from build123d import *

# Parameters (mm, degrees)
F1_DEPTH    = 80
F0_R        = 10
F2_DEPTH    = 40
F0_R_2      = 4
F3_DEPTH    = 5
F4_SIZE     = 2
F5_T1_DEPTH = 43.847334297


# Not quite as in the source:
# - a fillet or chamfer that OpenCascade refuses, or shapes differently, is made with other operations: its cross-section is extruded or revolved along the edge and cut away or added


with BuildPart() as f1:
    # F0 (on Top) → F1 (new body)
    with BuildSketch(Plane.XY):
        with BuildLine():
            ThreePointArc((26.9229627936, -13.2345787395), (29.220616727, -6.7937881992), (30, 0))
            ThreePointArc((30, 0), (29.220616727, 6.7937881992), (26.9229627936, 13.2345787395))
            Line((26.9229627936, 13.2345787395), (18.2336879396, 8.2178235635))
            ThreePointArc((18.2336879396, 8.2178235635), (19.5534365112, 4.2027515515), (20, 0))
            ThreePointArc((20, 0), (19.5534365112, -4.2027515515), (18.2336879396, -8.2178235635))
            Line((18.2336879396, -8.2178235635), (26.9229627936, -13.2345787395))
        make_face()
    extrude(amount=F1_DEPTH)



with BuildPart() as f1b:
    # F0 (on Top) → F1, piece 2 (new body)
    with BuildSketch(Plane.XY):
        with BuildLine():
            Line((16.2336879396, 11.6819251786), (24.9229627936, 16.6986803547))
            ThreePointArc((24.9229627936, 16.6986803547), (15.21659411, 25.8545018071), (2.5, 29.8956518578))
            Line((2.5, 29.8956518578), (2.5, 19.843134833))
            ThreePointArc((2.5, 19.843134833), (10.2170984976, 17.1933387767), (16.2336879396, 11.6819251786))
        make_face()
    extrude(amount=F1_DEPTH)


with BuildPart() as f1c:
    # F0 (on Top) → F1, piece 3 (new body)
    with BuildSketch(Plane.XY):
        with BuildLine():
            ThreePointArc((2.5, -29.8956518578), (15.21659411, -25.8545018071), (24.9229627936, -16.6986803547))
            Line((24.9229627936, -16.6986803547), (16.2336879396, -11.6819251786))
            ThreePointArc((16.2336879396, -11.6819251786), (10.2170984976, -17.1933387767), (2.5, -19.843134833))
            Line((2.5, -19.843134833), (2.5, -29.8956518578))
        make_face()
    extrude(amount=F1_DEPTH)


with BuildPart() as f1d:
    # F0 (on Top) → F1, piece 4 (new body)
    with BuildSketch(Plane.XY):
        with BuildLine():
            Line((-2.5, 19.843134833), (-2.5, 29.8956518578))
            ThreePointArc((-2.5, 29.8956518578), (-15.21659411, 25.8545018071), (-24.9229627936, 16.6986803547))
            Line((-24.9229627936, 16.6986803547), (-16.2336879396, 11.6819251786))
            ThreePointArc((-16.2336879396, 11.6819251786), (-10.2170984976, 17.1933387767), (-2.5, 19.843134833))
        make_face()
    extrude(amount=F1_DEPTH)


with BuildPart() as f1e:
    # F0 (on Top) → F1, piece 5 (new body)
    with BuildSketch(Plane.XY):
        with BuildLine():
            ThreePointArc((-24.9229627936, -16.6986803547), (-15.21659411, -25.8545018071), (-2.5, -29.8956518578))
            Line((-2.5, -29.8956518578), (-2.5, -19.843134833))
            ThreePointArc((-2.5, -19.843134833), (-10.2170984976, -17.1933387767), (-16.2336879396, -11.6819251786))
            Line((-16.2336879396, -11.6819251786), (-24.9229627936, -16.6986803547))
        make_face()
    extrude(amount=F1_DEPTH)


with BuildPart() as f1f:
    # F0 (on Top) → F1, piece 6 (new body)
    with BuildSketch(Plane.XY):
        with BuildLine():
            Line((-18.2336879396, 8.2178235635), (-26.9229627936, 13.2345787395))
            ThreePointArc((-26.9229627936, 13.2345787395), (-30, 0), (-26.9229627936, -13.2345787395))
            Line((-26.9229627936, -13.2345787395), (-18.2336879396, -8.2178235635))
            ThreePointArc((-18.2336879396, -8.2178235635), (-20, 0), (-18.2336879396, 8.2178235635))
        make_face()
    extrude(amount=F1_DEPTH)


with BuildPart() as f1_1:
    add(f1.part)

    add(f1b.part)  # F2 merges F1b

    add(f1c.part)  # F2 merges F1c

    add(f1d.part)  # F2 merges F1d

    add(f1e.part)  # F2 merges F1e

    add(f1f.part)  # F2 merges F1f
    # F0 (on Top) → F2 (join)
    with BuildSketch(Plane.XY):
        with BuildLine():
            Line((18.2336879396, 8.2178235635), (26.9229627936, 13.2345787395))
            ThreePointArc((26.9229627936, 13.2345787395), (25.9807621135, 15), (24.9229627936, 16.6986803547))
            Line((24.9229627936, 16.6986803547), (16.2336879396, 11.6819251786))
            ThreePointArc((16.2336879396, 11.6819251786), (17.3205080757, 10), (18.2336879396, 8.2178235635))
        make_face()
        with BuildLine():
            ThreePointArc((24.9229627936, -16.6986803547), (25.9807621135, -15), (26.9229627936, -13.2345787395))
            Line((26.9229627936, -13.2345787395), (18.2336879396, -8.2178235635))
            ThreePointArc((18.2336879396, -8.2178235635), (17.3205080757, -10), (16.2336879396, -11.6819251786))
            Line((16.2336879396, -11.6819251786), (24.9229627936, -16.6986803547))
        make_face()
        with BuildLine():
            ThreePointArc((20, 0), (19.5534365112, 4.2027515515), (18.2336879396, 8.2178235635))
            ThreePointArc((18.2336879396, 8.2178235635), (17.3205080757, 10), (16.2336879396, 11.6819251786))
            ThreePointArc((16.2336879396, 11.6819251786), (10.2170984976, 17.1933387767), (2.5, 19.843134833))
            ThreePointArc((2.5, 19.843134833), (0, 20), (-2.5, 19.843134833))
            ThreePointArc((-2.5, 19.843134833), (-10.2170984976, 17.1933387767), (-16.2336879396, 11.6819251786))
            ThreePointArc((-16.2336879396, 11.6819251786), (-17.3205080757, 10), (-18.2336879396, 8.2178235635))
            ThreePointArc((-18.2336879396, 8.2178235635), (-20, 0), (-18.2336879396, -8.2178235635))
            ThreePointArc((-18.2336879396, -8.2178235635), (-17.3205080757, -10), (-16.2336879396, -11.6819251786))
            ThreePointArc((-16.2336879396, -11.6819251786), (-10.2170984976, -17.1933387767), (-2.5, -19.843134833))
            ThreePointArc((-2.5, -19.843134833), (0, -20), (2.5, -19.843134833))
            ThreePointArc((2.5, -19.843134833), (10.2170984976, -17.1933387767), (16.2336879396, -11.6819251786))
            ThreePointArc((16.2336879396, -11.6819251786), (17.3205080757, -10), (18.2336879396, -8.2178235635))
            ThreePointArc((18.2336879396, -8.2178235635), (19.5534365112, -4.2027515515), (20, 0))
        make_face()
        Circle(F0_R, mode=Mode.SUBTRACT)
        with BuildLine():
            Line((2.5, 19.843134833), (2.5, 29.8956518578))
            ThreePointArc((2.5, 29.8956518578), (0, 30), (-2.5, 29.8956518578))
            Line((-2.5, 29.8956518578), (-2.5, 19.843134833))
            ThreePointArc((-2.5, 19.843134833), (0, 20), (2.5, 19.843134833))
        make_face()
        with BuildLine():
            ThreePointArc((-2.5, -29.8956518578), (0, -30), (2.5, -29.8956518578))
            Line((2.5, -29.8956518578), (2.5, -19.843134833))
            ThreePointArc((2.5, -19.843134833), (0, -20), (-2.5, -19.843134833))
            Line((-2.5, -19.843134833), (-2.5, -29.8956518578))
        make_face()
        with BuildLine():
            Line((-16.2336879396, 11.6819251786), (-24.9229627936, 16.6986803547))
            ThreePointArc((-24.9229627936, 16.6986803547), (-25.9807621135, 15), (-26.9229627936, 13.2345787395))
            Line((-26.9229627936, 13.2345787395), (-18.2336879396, 8.2178235635))
            ThreePointArc((-18.2336879396, 8.2178235635), (-17.3205080757, 10), (-16.2336879396, 11.6819251786))
        make_face()
        with BuildLine():
            ThreePointArc((-26.9229627936, -13.2345787395), (-25.9807621135, -15), (-24.9229627936, -16.6986803547))
            Line((-24.9229627936, -16.6986803547), (-16.2336879396, -11.6819251786))
            ThreePointArc((-16.2336879396, -11.6819251786), (-17.3205080757, -10), (-18.2336879396, -8.2178235635))
            Line((-18.2336879396, -8.2178235635), (-26.9229627936, -13.2345787395))
        make_face()
    extrude(amount=F2_DEPTH)

    # F0 (on Top) → F3 (join)
    with BuildSketch(Plane.XY):
        Circle(F0_R)
        Circle(F0_R_2, mode=Mode.SUBTRACT)
    extrude(amount=F3_DEPTH)

    # F4
    f4_edges = [f1_1.edges().sort_by_distance(p)[0] for p in [
        (-20.578325, 14.190303, 80),
        (-22.578325, 10.726201, 80),
        (-22.578325, -10.726201, 80),
        (-20.578325, -14.190303, 80),
        (20.578325, -14.190303, 80),
        (22.578325, -10.726201, 80),
        (22.578325, 10.726201, 80),
        (20.578325, 14.190303, 80),
        (-2.5, 24.869393, 80),
        (2.5, 24.869393, 80),
        (2.5, -24.869393, 80),
        (-2.5, -24.869393, 80),
    ]]
    chamfer(f4_edges, length=F4_SIZE)

    # F5: fillet of radius 2 on 6 edges, made by hand

    # F5_s2 → F5_t1 (cut)
    with BuildSketch(Plane.XY.offset(40)):
        with BuildLine():
            ThreePointArc((-2.5, 27.6360272109), (-3.2044030609, 29.1596507114), (-4.8214285714, 29.6100291545))
            ThreePointArc((-4.8214285714, 29.6100291545), (-3.6634988964, 29.7754727223), (-2.5, 29.8956518578))
            Line((-2.5, 29.8956518578), (-2.5, 27.6360272109))
        make_face()
        with BuildLine():
            ThreePointArc((4.8214285714, 29.6100291545), (3.2044030609, 29.1596507114), (2.5, 27.6360272109))
            Line((2.5, 27.6360272109), (2.5, 29.8956518578))
            ThreePointArc((2.5, 29.8956518578), (3.6634988964, 29.7754727223), (4.8214285714, 29.6100291545))
        make_face()
        with BuildLine():
            ThreePointArc((-4.8214285714, -29.6100291545), (-3.2044030609, -29.1596507114), (-2.5, -27.6360272109))
            Line((-2.5, -27.6360272109), (-2.5, -29.8956518578))
            ThreePointArc((-2.5, -29.8956518578), (-3.6634988964, -29.7754727223), (-4.8214285714, -29.6100291545))
        make_face()
        with BuildLine():
            ThreePointArc((4.8214285714, -29.6100291545), (3.2044030609, -29.1596507114), (2.5, -27.6360272109))
            Line((2.5, -27.6360272109), (2.5, -29.8956518578))
            ThreePointArc((2.5, -29.8956518578), (3.6634988964, -29.7754727223), (4.8214285714, -29.6100291545))
        make_face()
    extrude(amount=F5_T1_DEPTH, mode=Mode.SUBTRACT)


solid = f1_1.part
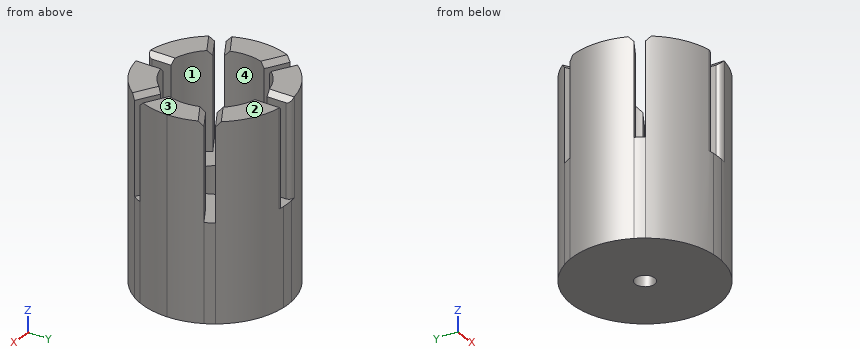
Here's how the part is built. I have some questions about the finished solid (model axes, mm). Face numbers are marked on the shaded views. A direction names the side the tool comes from. Round coordinates to 2 decimals unless told otherwise and drop trailing zeros. Loops run counter-clockwise (first coordinate to the right, second up) from the corner with the lowest first, then second, coordinate; pieces in that order, holes last.
1. For P1, Ø1, axis at y = 4.5, z = 29, coming from the -X side; P2, Ø6, axis at x = -4.5, y = -2.5, coming from the +Z side; P3, Ø2.5, axis at y = -22.5, z = 59, coming from the -X side, each with a flat end and sliding along its axis, tell me the tip position at first contact or that it passes through.
Answer list:
P1: stops at x = -29.73
P2: stops at z = 5
P3: stops at x = -21.18
2. If we section it at B-B on z = 49: Write out the boundary of the cut face in (x, y).
Answer list:
outline: (-26.92, -13.23) - (-18.23, -8.22) arc R20 cw to (-18.23, 8.22) - (-26.92, 13.23) arc R30 ccw to start; (-24.92, -16.7) arc R30 ccw to (-4.82, -29.61) arc R2 ccw to (-2.5, -27.64) - (-2.5, -19.84) arc R20 cw to (-16.23, -11.68) - close; (-24.92, 16.7) - (-16.23, 11.68) arc R20 cw to (-2.5, 19.84) - (-2.5, 27.64) arc R2 ccw to (-4.82, 29.61) arc R30 ccw to start; (2.5, -27.64) arc R2 ccw to (4.82, -29.61) arc R30 ccw to (24.92, -16.7) - (16.23, -11.68) arc R20 cw to (2.5, -19.84) - close; (2.5, 19.84) arc R20 cw to (16.23, 11.68) - (24.92, 16.7) arc R30 ccw to (4.82, 29.61) arc R2 ccw to (2.5, 27.64) - close; (18.23, -8.22) - (26.92, -13.23) arc R30 ccw to (26.92, 13.23) - (18.23, 8.22) arc R20 cw to start
3. If we section it at C-C on y = 21: Write out the boundary of the cut face in (x, z).
Answer list:
outline: (-21.42, 0) - (21.42, 0) - (21.42, 80) - (4.5, 80) - (2.5, 78) - (2.5, 40) - (-2.5, 40) - (-2.5, 78) - (-4.5, 80) - (-21.42, 80) - close
4. If we section it at A-A on x = 0: Write out the boundary of the cut face in (y, z), plus the area to 3 significant figures.
Answer list:
outline: (-30, 0) - (-4, 0) - (-4, 5) - (-10, 5) - (-10, 40) - (-30, 40) - close; (4, 0) - (30, 0) - (30, 40) - (10, 40) - (10, 5) - (4, 5) - close
area: 1,660 mm2
5. Which directions (+Z, -Z, +X, -X, +Y, -Y) give clear straight access to the entire face, cutting with the end or side of a thin tool? Please do the marked faces 3 and 4.
Answer list:
face 3: +Z, +X, -X, +Y, -Y
face 4: +Z
6. If we section it at D-D on x = 8: Write out the boundary of the cut face in (y, z).
Answer list:
outline: (-28.91, 0) - (28.91, 0) - (28.91, 80) - (18.33, 80) - (18.33, 40) - (6, 40) - (6, 5) - (-6, 5) - (-6, 40) - (-18.33, 40) - (-18.33, 80) - (-28.91, 80) - close
7. If I drill on line 1 along X through (y, z) = (-26, 19); line 2 along X through (y, z) = (-7.5, 10); line 3 along Z through (x, y) = (6, 15.5), over which ranges is the centre line in solid material (lowest first)?
Answer list:
line 1: x = -14.97 to 14.97
line 2: x = -29.05 to -6.61, 6.61 to 29.05
line 3: z = 0 to 40
8. We'd pull the mould along X, two halves only. Please class the marked faces 1 and 2: +X half, -X half, draft (parallel to the pull), parting line (faces both ways), or undercut.
Answer list:
face 1: undercut
face 2: draft
